Job drawing, mm, ordinate dimensions from the low corner. One solid piece. A direction names the side the tool comes from. Coordinates: 2 decimals unless noted, no trailing zeros. Write each loop counter-clockwise with the first axis right and the second up, starting at its lowest first coordinate (ties: lowest second). Pieces come first, ordered by that corner, then holes.
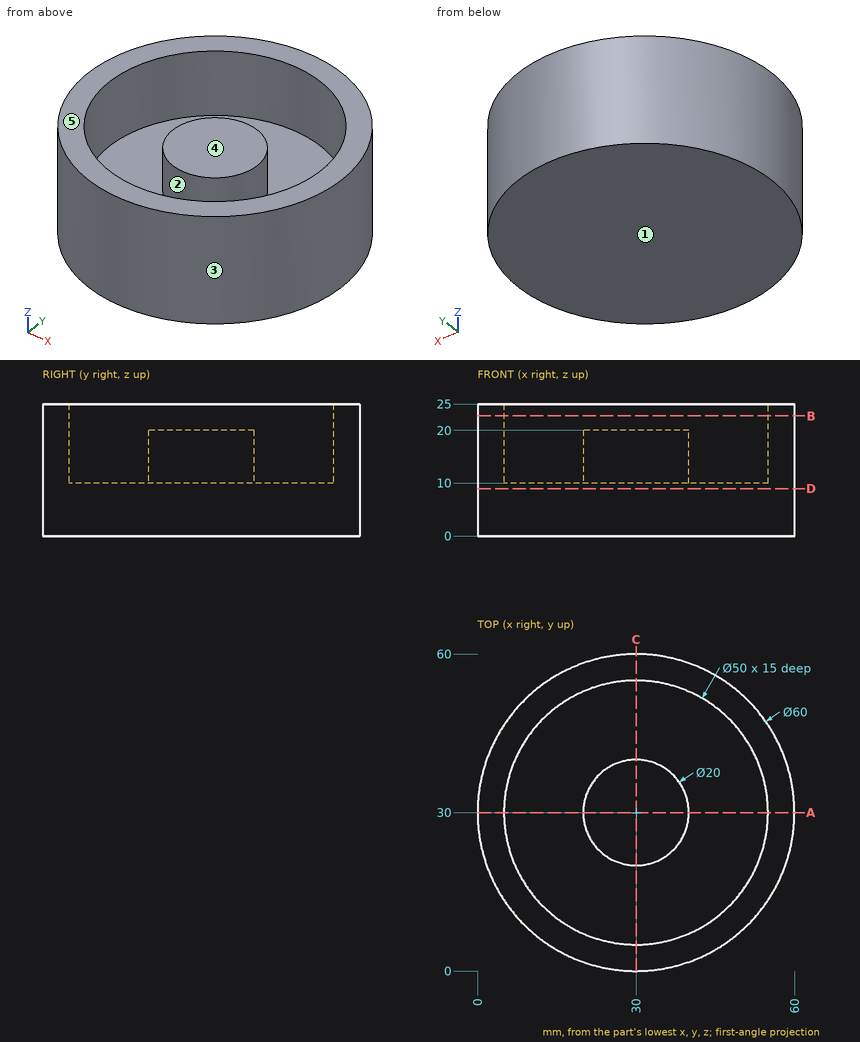
1. Saw through at D-D on z = 9. List the corners of the cut face in (x, y).
Computed values:
outline: circle Ø60 at (30, 30)
2. Flat gauge pins, fed straight in: pin 1 (12 mm diameter, centred on x = 42.5, z = 3, fed in from +Y); pin 2 (8 mm diameter, centred on y = 23.5, z = 18, fed in from -X); pin 3 (1.5 mm diameter, centred on x = 36.5, z = 20.5, fed in from +Y). Where does each tip first touch, or does it go through?
Computed values:
pin 1: stops at y = 59.29
pin 2: stops at x = 0.1
pin 3: stops at y = 59.44
3. Saw through at A-A on y = 30. List the corners of the cut face in (x, z).
Computed values:
outline: (0, 0) - (60, 0) - (60, 25) - (55, 25) - (55, 10) - (40, 10) - (40, 20) - (20, 20) - (20, 10) - (5, 10) - (5, 25) - (0, 25) - close
4. Saw through at B-B on z = 22.75. List the corners of the cut face in (x, y), plus the area to 3 significant figures.
Computed values:
outline: circle Ø60 at (30, 30); hole circle Ø50 at (30, 30)
area: 864 mm2
5. 3-axis set-ups, long thin cutter, end or side, ignore diameter. For the marked faces 4 and 5: which of +Z, -Z, +X, -X, +Y, -Y reach the whole face in a straight line?
Computed values:
face 4: +Z
face 5: +Z, +X, -X, +Y, -Y
6. Probe line 1 along Y through (x, z) = (30, 19); line 2 along Y through (x, z) = (30, 21.75); line 3 along X through (y, z) = (32, 18). List the from-to ranges inside material, lowest first.
Computed values:
line 1: y = 0 to 5, 20 to 40, 55 to 60
line 2: y = 0 to 5, 55 to 60
line 3: x = 0.07 to 5.08, 20.2 to 39.8, 54.92 to 59.93
7. Mould opens along Y. For the marked faces 1, 2 and 3 say: +Y half, -Y half, draft (parallel to the pull), parting line (faces both ways), or undercut.
Computed values:
face 1: draft
face 2: undercut
face 3: parting line
